Check sheet for the modelled part. Datum: model origin and axes. Units: mm. Face numbers are marked on the shaded views. A direction names the side the tool comes from. Coordinates: 2 decimals unless noted, no trailing zeros. Loops run counter-clockwise (first coordinate to the right, second up) from the corner with the lowest first, then second, coordinate; pieces in that order, holes last. Notation, with made-up numbers: (66.5, 26.5) -> (123.5, 26.5) arc R18 ccw to (123.5, 46.5) -> close; hole circle Ø6 at (4.25, 63.25). An arc over 180 degrees is marked (long way). Use CSV: the item, a comma, the result in double quotes. Start each with the question number.
1. Set-up check for the marked faces 4, 5 and 6: record each of +Z, -Z, +X, -X, +Y, -Y from which the full face is reachable in a straight line by a thin tool's end or side.
2. Sectioned sample at A-A, the plane x = 25. Record the cut outline in (y, z), and give its area (3 significant figures).
3. Thickness scan on L1, parallel to X at y = 2, z = 10; L2, parallel to Z at x = -13, y = 0; L3, parallel to Z at x = 24.5, y = 5. Record the ranges inside material, lowest first.
4. Sectioned sample at C-C, the plane y = 6. Record the cut outline in (x, z), and give its area (3 significant figures).
5. Gauge pin test, flat ends, axial feed: pin 1 (12 mm diameter, centred on x = 18, y = -2.5, fed in from -Z); pin 2 (1 mm diameter, centred on y = 5, z = -15, fed in from +X); pin 3 (6 mm diameter, centred on x = -20, y = 7.5, fed in from -Z). Record the tip position at first contact, or that the pin passes through.
6. Release check for a two-part mould opening along Y. For the marked faces 1, 2 and 3 record: pulls with the +Y half, pulls with the -Y half, needs draft (parallel to the pull), parting line crosses it, or undercut.
7. Sectioned sample at D-D, the plane x = -25. Record the cut outline in (y, z).
8. Sectioned sample at B-B, the plane z = 10. Record the cut outline in (x, y), and give its area (3 significant figures).
```python
from build123d import *

# Parameters (mm, degrees)
SKIZZE1_R                       = 6.5
AUFSATZ_LINEAR_AUSTRAGEN1_DEPTH = 10
F_10_0MM_STIFTLOCH1_D           = 10
F_10_0MM_STIFTLOCH1_DEPTH       = 22
F_10_0MM_STIFTLOCH1_TIP         = 3.004303095
SCHNITT_LINEAR_AUSTRAGEN2_DEPTH = 49.548944376
FASE1_SIZE                      = 5


with BuildPart() as part:
    # Skizze1 → Aufsatz-Linear austragen1 (new, symmetric)
    with BuildSketch(Plane(origin=(0, 0, 0), x_dir=(1, 0, 0), z_dir=(0, 1, 0))):
        Polygon((-40, -24), (40, -24), (40, 4), (-1, 4), (-1, 24), (-40, 24), align=None)
        with Locations(Location((-25, -10, 0), (0, 0, 270))):
            Circle(SKIZZE1_R, mode=Mode.SUBTRACT)
        with Locations(Location((25, -10, 0), (0, 0, 270))):
            Circle(SKIZZE1_R, mode=Mode.SUBTRACT)
    extrude(amount=AUFSATZ_LINEAR_AUSTRAGEN1_DEPTH, both=True)

    # Ø10.0mm Stiftloch1
    with Locations(Plane(origin=(-1, 0, 0), x_dir=(0, 0, -1), z_dir=(1, 0, 0))):
        with Locations((15, 0)):
            Hole(F_10_0MM_STIFTLOCH1_D / 2, depth=F_10_0MM_STIFTLOCH1_DEPTH)
            with Locations((0, 0, -(F_10_0MM_STIFTLOCH1_DEPTH + F_10_0MM_STIFTLOCH1_TIP / 2))):  # 118° drill point
                Cone(0, F_10_0MM_STIFTLOCH1_D / 2, F_10_0MM_STIFTLOCH1_TIP, mode=Mode.SUBTRACT)

    # Skizze5 → Schnitt-Linear austragen2 (cut, through all)
    with BuildSketch(Plane(origin=(-1, 0, 0), x_dir=(0, 0, -1), z_dir=(1, 0, 0))):
        with BuildLine():
            Line((14, 10), (26, 10))
            Line((26, 10), (26, -10))
            Line((26, -10), (14, -10))
            ThreePointArc((14, -10), (24, 0), (14, 10))
        make_face()
    extrude(amount=-SCHNITT_LINEAR_AUSTRAGEN2_DEPTH, mode=Mode.SUBTRACT)

    # Fase1
    fase1_edges = [part.edges().sort_by_distance(p)[0] for p in [
        (19.5, 10, -4),
        (0, 10, 24),
    ]]
    chamfer(fase1_edges, length=FASE1_SIZE)


solid = part.part
```
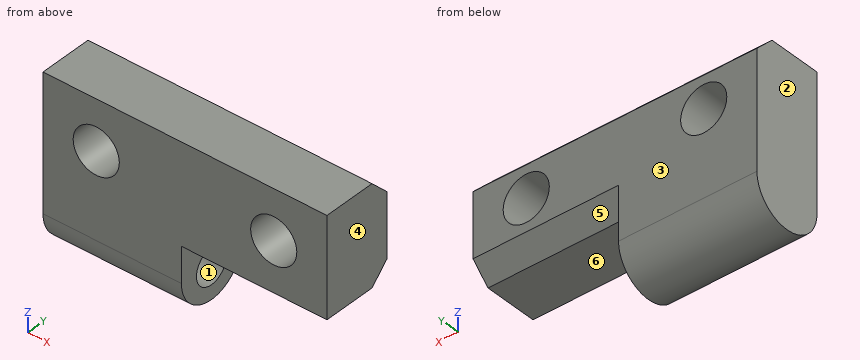
Completed:
1,face 4,"+Z, -Z, +X, +Y, -Y"
1,face 5,"-Z, +X, +Y"
1,face 6,"-Z, +X, +Y, -Y"
2,outline,"(-10, -4) -> (5, -4) -> (10, 1) -> (10, 3.5) -> (-10, 3.5) -> close; (-10, 16.5) -> (10, 16.5) -> (10, 19) -> (5, 24) -> (-10, 24) -> close"
2,area,"275 mm²"
3,L1,"-40 to -31.5, -18.5 to 18.5, 31.5 to 40"
3,L2,"-24 to -20, -10 to 24"
3,L3,"-4 to 3.52, 16.48 to 24"
4,outline,"(-40, -22) -> (-1, -22) -> (-1, -3) -> (40, -3) -> (40, 23) -> (-40, 23) -> close; hole circle Ø13 at (-25, 10); hole circle Ø13 at (25, 10)"
4,area,"2,560 mm²"
5,pin 1,"z = -4"
5,pin 2,"x = -1"
5,pin 3,"z = -22.93"
6,face 1,"undercut"
6,face 2,"needs draft"
6,face 3,"pulls with the +Y half"
7,outline,"(-10, -14) arc R10 ccw to (10, -14) -> (10, 3.5) -> (-10, 3.5) -> close; (-10, 16.5) -> (10, 16.5) -> (10, 19) -> (5, 24) -> (-10, 24) -> close; hole circle Ø3.34 at (0, -15)"
8,outline,"(-40, -10) -> (-31.5, -10) -> (-31.5, 10) -> (-40, 10) -> close; (-18.5, -10) -> (18.5, -10) -> (18.5, 10) -> (-18.5, 10) -> close; (31.5, -10) -> (40, -10) -> (40, 10) -> (31.5, 10) -> close"
8,area,"1,080 mm²"
